Geometry check sheet. Reference: the model listing, model coordinates, mm. Coordinates: 2 decimals unless noted, no trailing zeros. Loops run counter-clockwise (first coordinate to the right, second up) from the corner with the lowest first, then second, coordinate; pieces in that order, holes last. Notation, with made-up numbers: M -22,-16.75 L 21,-16.75 A13 ccw 21,4.25 Z; hole C -8,34 d4. An arc over 180 degrees is marked long. Use CSV: the item, a comma, the result in double quotes.
```python
from build123d import *

# Parameters (mm, degrees)
ESQUISSE1_W                              = 57
ESQUISSE1_H                              = 10
BOSS_EXTRU_1_DEPTH                       = 10
FRAISAGE_POUR_VIS_T_TE_FRAIS_E_6_2_COUNT = 2
FRAISAGE_POUR_VIS_T_TE_FRAIS_E_6_2_PITCH = 29
ESQUISSE8_R                              = 1.55
ENL_V_MAT_EXTRU_1_DEPTH                  = 5


with BuildPart() as part:
    # Esquisse1 → Boss.-Extru.1 (new body)
    with BuildSketch(Plane.XY):
        with Locations((0, -22.219493411)):
            Rectangle(ESQUISSE1_W, ESQUISSE1_H)
    extrude(amount=BOSS_EXTRU_1_DEPTH)

    # Esquisse6 → Fraisage pour vis à tête fraisée à 6 pans creux M31 (revolve, cut)
    with BuildSketch(Plane(origin=(-14.5, -22.219493411, 10), x_dir=(0, -1, 0), z_dir=(1, 0, 0))):
        Polygon((0, 0), (0, 10), (1.6, 10), (1.6, 1.7), (2.9, 0.4), (2.9, 0), align=None)
    fraisage_pour_vis_t_te_frais_e_6_pan = revolve(axis=Axis((-14.5, -22.219493411, 16.35), (0, 0, -1)), mode=Mode.SUBTRACT)

    # Fraisage pour vis _ t_te frais_e _ 6 2: Fraisage pour vis à tête fraisée à 6 pans creux M31 ×2
    with Locations(*[(i * FRAISAGE_POUR_VIS_T_TE_FRAIS_E_6_2_PITCH, 0, 0) for i in range(1, FRAISAGE_POUR_VIS_T_TE_FRAIS_E_6_2_COUNT)]):
        add(fraisage_pour_vis_t_te_frais_e_6_pan, mode=Mode.SUBTRACT)

    # Esquisse8 → Enlèv. mat.-Extru.1 (cut)
    with BuildSketch(Plane(origin=(0, 0, 0), x_dir=(-1, 0, 0), z_dir=(0, 0, -1))):
        with Locations((-23.5, -22.219493411)):
            Circle(ESQUISSE8_R)
    enl_v_mat_extru_1 = extrude(amount=-ENL_V_MAT_EXTRU_1_DEPTH, mode=Mode.SUBTRACT)

    # Symétrie1: Enlèv. mat.-Extru.1 across plane
    add(enl_v_mat_extru_1.mirror(Plane(origin=(0, 0, 0), x_dir=(0, 0, 1), z_dir=(1, 0, 0))), mode=Mode.SUBTRACT)


solid = part.part
```
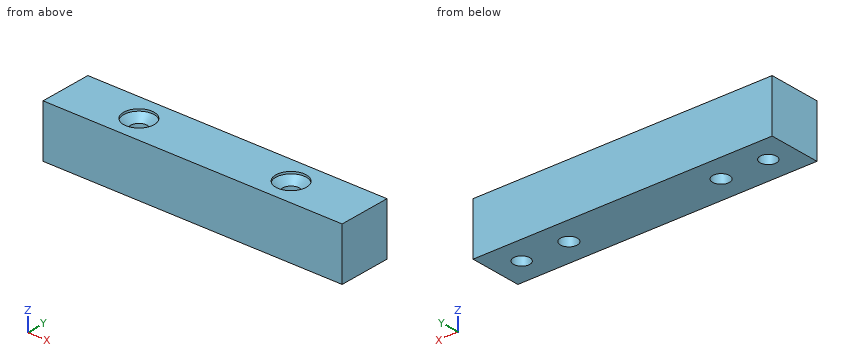
1. Thickness scan on line 1 (X direction, y = -24, z = 9.75); line 2 (X direction, y = -22, z = 8); line 3 (Y direction, x = 23.5, z = 3.8). Record the ranges inside material, lowest first. Write a range as [from, to].
The answers:
line 1,"[-28.5, -16.79], [-12.21, 12.21], [16.79, 28.5]"
line 2,"[-28.5, -16.08], [-12.92, 12.92], [16.08, 28.5]"
line 3,"[-27.22, -23.77], [-20.67, -17.22]"
2. Section check B-B, the plane z = 6. Record the cut outline in (x, y), plus the area to 3 significant figures.
The answers:
outline,"M -28.5,-27.22 L 28.5,-27.22 L 28.5,-17.22 L -28.5,-17.22 Z; hole C -14.5,-22.22 d3.2; hole C 14.5,-22.22 d3.2"
area,"554 mm^2"
3. Section check A-A, the plane x = 14.5. Record the cut outline in (y, z), plus the area to 3 significant figures.
The answers:
outline,"M -27.22,0 L -23.82,0 L -23.82,8.3 L -25.12,9.6 L -25.12,10 L -27.22,10 Z; M -20.62,0 L -17.22,0 L -17.22,10 L -19.32,10 L -19.32,9.6 L -20.62,8.3 Z"
area,"65.3 mm^2"
4. Section check C-C, the plane x = -23.5. Record the cut outline in (y, z).
The answers:
outline,"M -27.22,0 L -23.77,0 L -23.77,5 L -20.67,5 L -20.67,0 L -17.22,0 L -17.22,10 L -27.22,10 Z"
5. Gauge pin test, flat ends, axial feed: P1, Ø3, axis at x = -14.5, y = -22.22, coming from the -Z side; P2, Ø1.6, axis at x = 23.5, y = -22, coming from the -Z side; P3, Ø5, axis at x = 14.5, y = -22.22, coming from the +Z side. Record the tip position at first contact, or that the pin passes through.
The answers:
P1,"through"
P2,"z = 5"
P3,"z = 9.2"
6. Section check D-D, the plane z = 0.75. Record the cut outline in (x, y), plus the area to 3 significant figures.
The answers:
outline,"M -28.5,-27.22 L 28.5,-27.22 L 28.5,-17.22 L -28.5,-17.22 Z; hole C -23.5,-22.22 d3.1; hole C -14.5,-22.22 d3.2; hole C 14.5,-22.22 d3.2; hole C 23.5,-22.22 d3.1"
area,"539 mm^2"
